Geometry: see drawing. Coordinates: mm, zero at the bounding-box minimum. Give positions to 0.01 mm unless a question says otherwise; leave off trailing zeros. Loops run counter-clockwise (first coordinate to the right, second up) from the corner with the lowest first, then second, coordinate; pieces in that order, holes last. Notation, with made-up numbers: M 5.25,18.25 L 38.25,18.25 A22 ccw 38.25,34.25 Z; hole C 42.25,19.25 d5. An arc over 180 degrees is marked long. Put each result on its own line as item: value.
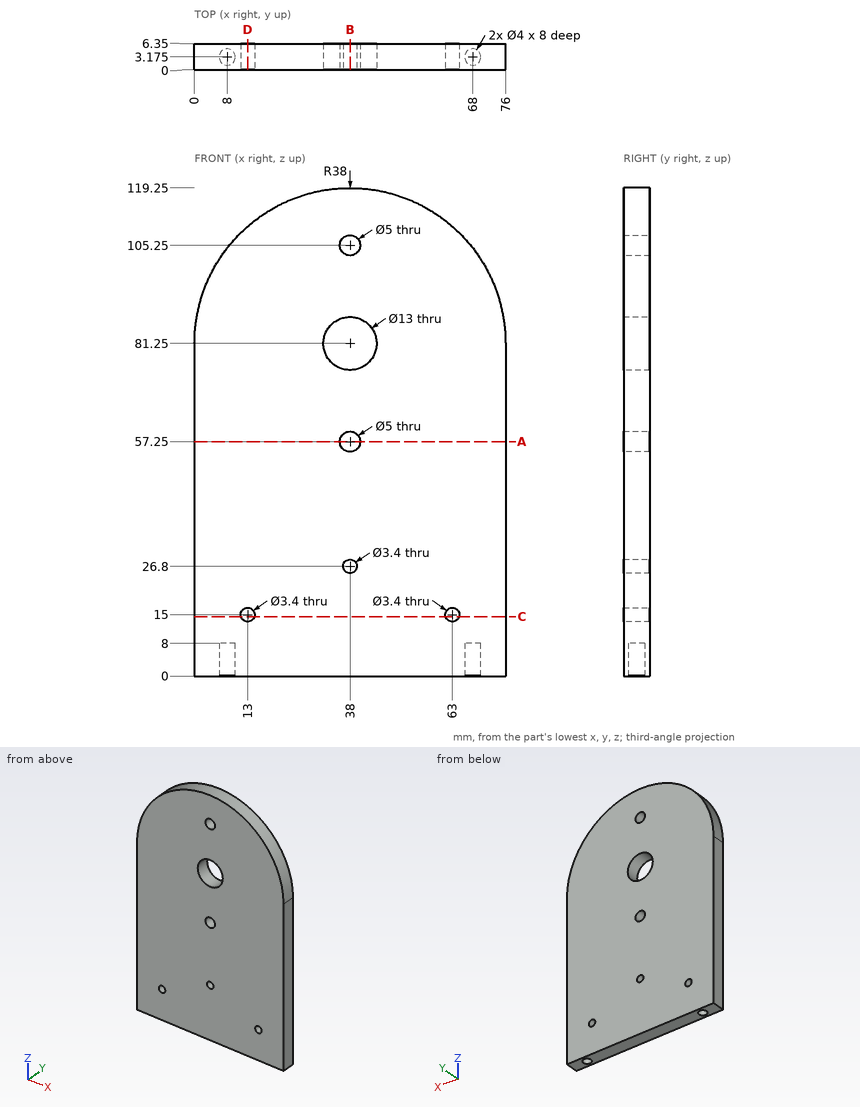
1. Material intervals for line 1 (X direction, y = 4.25, z = 81.25); line 2 (X direction, y = 3, z = 86); line 3 (Y direction, x = 68, z = 2.25) (3 decimals), sorted ascending. Write a range as from..to.
Found:
line 1: 0..31.5, 44.5..76
line 2: 0.3..33.56, 42.44..75.7
line 3: 0..1.175, 5.175..6.35
2. Section query C-C (z = 14.5). Output: boundary loops of the cut face in (x, y).
Found:
outline: M 0,0 L 11.38,0 L 11.38,6.35 L 0,6.35 Z; M 14.62,0 L 61.38,0 L 61.38,6.35 L 14.62,6.35 Z; M 64.62,0 L 76,0 L 76,6.35 L 64.62,6.35 Z
3. Section query D-D (x = 13). Output: boundary loops of the cut face in (y, z), plus the area to 3 significant figures.
Found:
outline: M 0,0 L 6.35,0 L 6.35,13.3 L 0,13.3 Z; M 0,16.7 L 6.35,16.7 L 6.35,109.87 L 0,109.87 Z
area: 676 mm^2
4. Contact query for flat-ended pins moving along their axis: P1, Ø3, axis at x = 38, z = 26.8, coming from the -Y side; P2, Ø2, axis at x = 15.5, y = 3, coming from the +Z side; P3, Ø2.5, axis at x = 68, y = 3.175, coming from the -Z side. Output: stop coordinate, or through.
Found:
P1: through
P2: z = 112.58
P3: z = 8
5. Section query B-B (x = 38). Output: boundary loops of the cut face in (y, z), plus the area to 3 significant figures.
Found:
outline: M 0,0 L 6.35,0 L 6.35,25.1 L 0,25.1 Z; M 0,28.5 L 6.35,28.5 L 6.35,54.75 L 0,54.75 Z; M 0,59.75 L 6.35,59.75 L 6.35,74.75 L 0,74.75 Z; M 0,87.75 L 6.35,87.75 L 6.35,102.75 L 0,102.75 Z; M 0,107.75 L 6.35,107.75 L 6.35,119.25 L 0,119.25 Z
area: 590 mm^2
6. Section query A-A (z = 57.25). Output: boundary loops of the cut face in (x, y), plus the area to 3 significant figures.
Found:
outline: M 0,0 L 35.5,0 L 35.5,6.35 L 0,6.35 Z; M 40.5,0 L 76,0 L 76,6.35 L 40.5,6.35 Z
area: 451 mm^2
